Here's how the part is built. I have some questions about the finished solid (model axes, mm). A direction names the side the tool comes from. Coordinates: 2 decimals unless noted, no trailing zeros. Write each loop counter-clockwise with the first axis right and the second up, starting at its lowest first coordinate (ties: lowest second). Pieces come first, ordered by that corner, then holes.
Item 1: For faces 1 (the face through (1, 1, -30)), 2 (the face through (-2.17, -9.76, 315.87)), which set-ups out of +Z, -Z, +X, -X, +Y, -Y let a thin tool reach every point of the face, with its end or its side?
Item 2: If we section it at C-C (z = 84): Please give me the cut outline in (x, y).
Item 3: If we section it at A-A (y = 0): Please give me the cut outline in (x, z), then the cut area to 4 significant figures.
Item 4: I'm going to push a flat-ended pin straight in: pin 1 Ø1.5 at (y, z) = (-3, 275.5) entering from +X. Where does the tip first touch, or does it pass through?
Item 5: If we section it at D-D (y = -73.5): Please give me the cut outline in (x, z) (3 decimals).
Item 6: If I drill on line 1 (Z direction, x = 80.5, y = 32.5); line 2 (Y direction, x = -1, z = 207); line 3 (X direction, y = -28, z = 23), over which ranges is the centre line in solid material (lowest first)?
from build123d import *

# Parameters (mm, degrees)
SKETCH1_R                = 88
BOSS_EXTRUDE3_DEPTH      = 25
SKETCH4_W                = 10.4719
SKETCH4_H                = 13.351164338
BOSS_EXTRUDE4_DEPTH      = 25
FILLET2_R                = 4
CIRPATTERN1_COUNT        = 30
FILLET2_OF_CIRPATTERN1_R = 4
SKETCH6_R                = 10
BOSS_EXTRUDE5_DEPTH      = 60
BOSS_EXTRUDE6_START      = 10
SKETCH7_R                = 10
BOSS_EXTRUDE6_DEPTH      = 10
SKETCH8_R                = 10
BOSS_EXTRUDE7_DEPTH      = 10
SKETCH9_R                = 10
BOSS_EXTRUDE8_DEPTH      = 25
SKETCH10_R               = 10
BOSS_EXTRUDE9_DEPTH      = 42.5
SKETCH12_R               = 12.5
CUT_EXTRUDE1_DEPTH       = 12
CUT_EXTRUDE2_START       = -55.5
SKETCH13_R               = 10
CUT_EXTRUDE2_DEPTH       = 55.5
SKETCH14_R               = 10
BOSS_EXTRUDE10_DEPTH     = 440
SKETCH15_R               = 105
BOSS_EXTRUDE12_DEPTH     = 25
BOSS_EXTRUDE13_START     = 30
SKETCH16_R               = 105
BOSS_EXTRUDE13_DEPTH     = 30
SKETCH17_R               = 10
BOSS_EXTRUDE14_DEPTH     = 50
SKETCH18_R               = 10
BOSS_EXTRUDE15_DEPTH     = 30


with BuildPart() as part:
    # Sketch1 → Boss-Extrude3 (new body)
    with BuildSketch(Plane.XY):
        Circle(SKETCH1_R)
    extrude(amount=BOSS_EXTRUDE3_DEPTH)

    # Sketch4 → Boss-Extrude4 (add)
    with BuildSketch(Plane.XY.offset(25)):
        with Locations((0, 93.324417831)):
            Rectangle(SKETCH4_W, SKETCH4_H)
    boss_extrude4 = extrude(amount=-BOSS_EXTRUDE4_DEPTH)

    # Fillet2
    fillet2_edges = [part.edges().sort_by_distance(p)[0] for p in [
        (5.23595, 100, 12.5),
        (0, 100, 0),
        (-5.23595, 100, 12.5),
        (0, 100, 25),
    ]]
    fillet(fillet2_edges, radius=FILLET2_R)

    # CirPattern1: Boss-Extrude4 ×30 about axis
    cirpattern1_axis = Axis((0, 0.317667884, 0), (0, 0, 1))
    for i in range(1, CIRPATTERN1_COUNT):
        add(boss_extrude4.rotate(cirpattern1_axis, i * 360 / CIRPATTERN1_COUNT))

    # Fillet2 of CirPattern1
    fillet2_of_cirpattern1_edges = [part.edges().sort_by_distance(p)[0] for p in [
        (-15.603590285, 98.910317096, 12.5),
        (-20.725122215, 97.821701879, 0),
        (-25.846654145, 96.733086661, 12.5),
        (-20.725122215, 97.821701879, 25),
        (-35.7611788, 93.511662322, 12.5),
        (-40.544457139, 91.382009596, 0),
        (-45.327735478, 89.252356869, 12.5),
        (-40.544457139, 91.382009596, 25),
        (-54.3558322, 84.039982796, 12.5),
        (-58.591804732, 80.962368605, 0),
        (-62.827777264, 77.884754413, 12.5),
        (-58.591804732, 80.962368605, 25),
        (-70.574874905, 70.909236365, 12.5),
        (-74.078409304, 67.018167216, 0),
        (-77.581943702, 63.127098067, 12.5),
        (-74.078409304, 67.018167216, 25),
        (-83.709456921, 54.693299655, 12.5),
        (-86.327431921, 50.158833942, 0),
        (-88.945406921, 45.624368229, 12.5),
        (-86.327431921, 50.158833942, 25),
        (-93.185533987, 36.100886913, 12.5),
        (-94.803531519, 31.121202547, 0),
        (-96.42152905, 26.14151818, 12.5),
        (-94.803531519, 31.121202547, 25),
        (-98.588956064, 15.944575793, 12.5),
        (-99.136261871, 10.737308875, 0),
        (-99.683567678, 5.530041957, 12.5),
        (-99.136261871, 10.737308875, 25),
        (-99.683567678, -4.894706189, 12.5),
        (-99.136261871, -10.101973107, 0),
        (-98.588956064, -15.309240025, 12.5),
        (-99.136261871, -10.101973107, 25),
        (-96.42152905, -25.506182413, 12.5),
        (-94.803531519, -30.485866779, 0),
        (-93.185533987, -35.465551145, 12.5),
        (-94.803531519, -30.485866779, 25),
        (-88.945406921, -44.989032461, 12.5),
        (-86.327431921, -49.523498174, 0),
        (-83.709456921, -54.057963887, 12.5),
        (-86.327431921, -49.523498174, 25),
        (-77.581943702, -62.491762299, 12.5),
        (-74.078409304, -66.382831448, 0),
        (-70.574874905, -70.273900597, 12.5),
        (-74.078409304, -66.382831448, 25),
        (-62.827777264, -77.249418645, 12.5),
        (-58.591804732, -80.327032837, 0),
        (-54.3558322, -83.404647029, 12.5),
        (-58.591804732, -80.327032837, 25),
        (-45.327735478, -88.617021102, 12.5),
        (-40.544457139, -90.746673828, 0),
        (-35.7611788, -92.876326554, 12.5),
        (-40.544457139, -90.746673828, 25),
        (-25.846654145, -96.097750894, 12.5),
        (-20.725122215, -97.186366111, 0),
        (-15.603590285, -98.274981329, 12.5),
        (-20.725122215, -97.186366111, 25),
        (-5.23595, -99.364664232, 12.5),
        (0, -99.364664232, 0),
        (5.23595, -99.364664232, 12.5),
        (0, -99.364664232, 25),
        (15.603590285, -98.274981329, 12.5),
        (20.725122215, -97.186366111, 0),
        (25.846654145, -96.097750894, 12.5),
        (20.725122215, -97.186366111, 25),
        (35.7611788, -92.876326554, 12.5),
        (40.544457139, -90.746673828, 0),
        (45.327735478, -88.617021102, 12.5),
        (40.544457139, -90.746673828, 25),
        (54.3558322, -83.404647029, 12.5),
        (58.591804732, -80.327032837, 0),
        (62.827777264, -77.249418645, 12.5),
        (58.591804732, -80.327032837, 25),
        (70.574874905, -70.273900597, 12.5),
        (74.078409304, -66.382831448, 0),
        (77.581943702, -62.491762299, 12.5),
        (74.078409304, -66.382831448, 25),
        (83.709456921, -54.057963887, 12.5),
        (86.327431921, -49.523498174, 0),
        (88.945406921, -44.989032461, 12.5),
        (86.327431921, -49.523498174, 25),
        (93.185533987, -35.465551145, 12.5),
        (94.803531519, -30.485866779, 0),
        (96.42152905, -25.506182413, 12.5),
        (94.803531519, -30.485866779, 25),
        (98.588956064, -15.309240025, 12.5),
        (99.136261871, -10.101973107, 0),
        (99.683567678, -4.894706189, 12.5),
        (99.136261871, -10.101973107, 25),
        (99.683567678, 5.530041957, 12.5),
        (99.136261871, 10.737308875, 0),
        (98.588956064, 15.944575793, 12.5),
        (99.136261871, 10.737308875, 25),
        (96.42152905, 26.14151818, 12.5),
        (94.803531519, 31.121202547, 0),
        (93.185533987, 36.100886913, 12.5),
        (94.803531519, 31.121202547, 25),
        (88.945406921, 45.624368229, 12.5),
        (86.327431921, 50.158833942, 0),
        (83.709456921, 54.693299655, 12.5),
        (86.327431921, 50.158833942, 25),
        (77.581943702, 63.127098067, 12.5),
        (74.078409304, 67.018167216, 0),
        (70.574874905, 70.909236365, 12.5),
        (74.078409304, 67.018167216, 25),
        (62.827777264, 77.884754413, 12.5),
        (58.591804732, 80.962368605, 0),
        (54.3558322, 84.039982796, 12.5),
        (58.591804732, 80.962368605, 25),
        (45.327735478, 89.252356869, 12.5),
        (40.544457139, 91.382009596, 0),
        (35.7611788, 93.511662322, 12.5),
        (40.544457139, 91.382009596, 25),
        (25.846654145, 96.733086661, 12.5),
        (20.725122215, 97.821701879, 0),
        (15.603590285, 98.910317096, 12.5),
        (20.725122215, 97.821701879, 25),
    ]]
    fillet(fillet2_of_cirpattern1_edges, radius=FILLET2_OF_CIRPATTERN1_R)

    # Sketch6 → Boss-Extrude5 (add)
    with BuildSketch(Plane.XY.offset(25)):
        Circle(SKETCH6_R)
    extrude(amount=BOSS_EXTRUDE5_DEPTH)

    # Sketch7 → Boss-Extrude6 (add)
    with BuildSketch(Plane(origin=(0, 0, 0), x_dir=(-1, 0, 0), z_dir=(0, 0, -1)).offset(BOSS_EXTRUDE6_START)):
        with Locations(Location((0, 0, 0), (0, 0, 180))):
            Circle(SKETCH7_R)
    extrude(amount=-BOSS_EXTRUDE6_DEPTH)

    # Sketch8 → Boss-Extrude7 (add)
    with BuildSketch(Plane.XY.offset(85)):
        Circle(SKETCH8_R)
    extrude(amount=BOSS_EXTRUDE7_DEPTH)

    # Sketch9 → Boss-Extrude8 (add)
    with BuildSketch(Plane.XY.offset(95)):
        Circle(SKETCH9_R)
    extrude(amount=BOSS_EXTRUDE8_DEPTH)

    # Sketch10 → Boss-Extrude9 (add)
    with BuildSketch(Plane.XY.offset(120)):
        Circle(SKETCH10_R)
    extrude(amount=BOSS_EXTRUDE9_DEPTH)

    # Sketch12 → Cut-Extrude1 (cut)
    with BuildSketch(Plane.XY.offset(162.5)):
        Circle(SKETCH12_R)
    extrude(amount=-CUT_EXTRUDE1_DEPTH, mode=Mode.SUBTRACT)

    # Sketch13 → Cut-Extrude2 (cut)
    with BuildSketch(Plane.XY.offset(150.5).offset(CUT_EXTRUDE2_START)):
        Circle(SKETCH13_R)
    extrude(amount=CUT_EXTRUDE2_DEPTH, mode=Mode.SUBTRACT)

    # Sketch14 → Boss-Extrude10 (add)
    with BuildSketch(Plane.XY.offset(95)):
        Circle(SKETCH14_R)
    extrude(amount=BOSS_EXTRUDE10_DEPTH)

    # Sketch15 → Boss-Extrude12 (add)
    with BuildSketch(Plane(origin=(0, 0, 0), x_dir=(-1, 0, 0), z_dir=(0, 0, -1))):
        Circle(SKETCH15_R)
    extrude(amount=-BOSS_EXTRUDE12_DEPTH)

    # Sketch16 → Boss-Extrude13 (add)
    with BuildSketch(Plane(origin=(0, 0, 0), x_dir=(-1, 0, 0), z_dir=(0, 0, -1)).offset(BOSS_EXTRUDE13_START)):
        Circle(SKETCH16_R)
    extrude(amount=-BOSS_EXTRUDE13_DEPTH)

    # Sketch17 → Boss-Extrude14 (add)
    with BuildSketch(Plane.XY.offset(535)):
        Circle(SKETCH17_R)
    extrude(amount=BOSS_EXTRUDE14_DEPTH)

    # Sketch18 → Boss-Extrude15 (add)
    with BuildSketch(Plane.XY.offset(585)):
        Circle(SKETCH18_R)
    extrude(amount=BOSS_EXTRUDE15_DEPTH)


solid = part.part
Answer list:
1. face 1: -Z, +X, -X, +Y, -Y
1. face 2: +Z
2. outline: circle Ø20 at (0, 0)
3. outline: (-105, -30) - (105, -30) - (105, 25) - (10, 25) - (10, 615) - (-10, 615) - (-10, 25) - (-105, 25) - close
3. area: 23,350 mm2
4. pin 1: stops at x = 9.74
5. outline: (-74.985, -30) - (74.985, -30) - (74.985, 25) - (-74.985, 25) - close
6. line 1: z = -30 to 25
6. line 2: y = -9.95 to 9.95
6. line 3: x = -101.2 to 101.2
